Autodesk Inventor part; units mm, degrees
ref_plane "YZ Plane" through (0, 0, 0) normal (1, 0, 0) x (0, 1, 0)
ref_plane "XZ Plane" through (0, 0, 0) normal (0, 1, 0) x (-1, 0, 0)
ref_plane "XY Plane" through (0, 0, 0) normal (0, 0, 1) x (1, 0, 0)
sketch "Sketch1" plane through (0, 0, 0) normal (0, 1, 0) x (-1, 0, 0)
  line L0 (0, 0) -> (22.8, 0)
  line L1 (22.8, 0) -> (22.8, -12.6)
  line L2 (22.8, -12.6) -> (0, -12.6)
  line L3 (0, -12.6) -> (0, 0)
  dimension "d0" = 22.8
  dimension "d1" = 12.6
extrude "Extrusion1" add sketch "Sketch1" along normal blind 16
sketch "Sketch2" plane through (0, 16, 0) normal (0, 1, 0) x (1, 0, 0)
  line L0 (0, 0) -> (4.85, 0)
  line L1 (4.85, 0) -> (4.85, 12.6)
  line L2 (0, 12.6) -> (-22.8, 12.6)
  line L3 (4.85, 12.6) -> (-22.8, 12.6)
  line L4 (-22.8, 12.6) -> (-27.65, 12.6)
  line L5 (-27.65, 12.6) -> (-27.65, 0)
  line L6 (-27.65, 0) -> (4.85, 0)
  line L7 (-22.8, 0) -> (0, 0)
  dimension "d4" = 4.85
  dimension "d5" = 4.85
extrude "Extrusion2" add sketch "Sketch2" along normal blind 2
sketch "Sketch3" plane through (0, 18, 0) normal (0, 1, 0) x (1, 0, 0)
  line L0 (-27.65, 0) -> (-22.8, 0)
  line L1 (0, 0) -> (0, 12.6)
  line L2 (-22.8, 0) -> (0, 0)
  line L3 (0, 0) -> (0, 12.6)
  line L4 (0, 12.6) -> (-22.8, 12.6)
  line L5 (-22.8, 12.6) -> (-22.8, 0)
extrude "Extrusion3" add sketch "Sketch3" along normal blind 1
sketch "Sketch4" plane through (0, 18, 0) normal (0, 1, 0) x (1, 0, 0)
  line L0 (-27.65, 12.6) -> (-27.65, 0)
  circle A0 centre (-26.09, 6.3) radius 1
  circle A1 centre (3.29, 6.3) radius 1
  line L1 (4.85, 0) -> (4.85, 12.6)
  point P0 (0, 0)
  dimension "d11" = 1.56
  dimension "d12" = 2
  dimension "d13" = 2
  dimension "d14" = 1.56
extrude "Extrusion4" cut sketch "Sketch4" against normal through all
sketch "Sketch5" plane through (-27.65, 18, -12.6) normal (0, 1, 0) x (1, 0, 0)
  point P0 (27.65, -12.6)
sketch "Sketch6" plane through (-27.65, 18, -12.6) normal (0, 1, 0) x (1, 0, 0)
  line L0 (4.85, 0) -> (0, 0)
  line L1 (4.85, 0) -> (27.65, 0)
  line L2 (27.65, 0) -> (27.65, -12.6)
  line L3 (27.65, -12.6) -> (4.85, -12.6)
  line L4 (4.85, -12.6) -> (4.85, 0)
extrude "Extrusion5" add sketch "Sketch6" along normal blind 4.4
sketch "Sketch7" plane through (-27.65, 22.4, -12.6) normal (0, 1, 0) x (1, 0, 0)
  circle A0 centre (21.35, -6.3) radius 6.3
  line L0 (27.65, -12.6) -> (4.85, -12.6)
  line L1 (27.65, -12.6) -> (27.65, 0)
  circle A1 centre (14.1367, -6.3) radius 3
  dimension "d22" = 6.3
  dimension "d23" = 6
extrude "Extrusion6" add sketch "Sketch7" along normal blind 4.3 contours A0 A1 | A1 A0 picked at (24.082, -5.787) picked at (15.7711, -6.9546)
sketch "Sketch8" plane through (-27.65, 22.4, -12.6) normal (0, 1, 0) x (1, 0, 0)
  circle A0 centre (14.5284, -6.3) radius 3
  point P0 (27.65, -12.6)
  dimension "d26" = 6
extrude "Extrusion7" add sketch "Sketch8" along normal blind 4.3
sketch "Sketch9" plane through (-27.65, 26.7, -12.6) normal (0, 1, 0) x (1, 0, 0)
  arc A0 (15.6897, -9.0661) -> (15.6897, -3.5339) centre (21.35, -6.3) ccw
  circle A1 centre (21.35, -6.3) radius 2
  point P0 (27.65, -12.6)
  dimension "d29" = 4
extrude "Extrusion8" add sketch "Sketch9" along normal blind 4
properties part number "SG92R"
Verification items for the finished model (mm, model axes). A direction names the side the tool comes from. Round coordinates to 2 decimals unless told otherwise and drop trailing zeros. Write each loop counter-clockwise with the first axis right and the second up, starting at its lowest first coordinate (ties: lowest second). Pieces come first, ordered by that corner, then holes.
(1) Section check D-D (x = -10.5). Enter the section's corners in (y, z), plus the area to 3 significant figures.
Returned:
outline: (0, -12.6) - (22.4, -12.6) - (22.4, -11) - (26.7, -11) - (26.7, -1.6) - (22.4, -1.6) - (22.4, 0) - (0, 0) - close
area: 323 mm2
(2) Mould release check, pull along Z, two halves, no side actions. Record for faces 1 (the cylindrical face through (3.16, 17.01, -7.29)), 2 (the cylindrical face through (-25.136, 17.014, -6.6)), 3 (the flat face through (-1.5, 22.4, -11.3)), 4 (the cylindrical face through (-6.734, 28.672, -8.252)): pulls with the +Z half, pulls with the -Z half, needs draft (parallel to the pull), parting line crosses it, or undercut.
Returned:
face 1: undercut
face 2: undercut
face 3: needs draft
face 4: parting line crosses it
(3) Section check B-B (y = 17.5). Enter the section's corners in (x, z), plus the area to 3 significant figures.
Returned:
outline: (-27.65, -12.6) - (4.85, -12.6) - (4.85, 0) - (-27.65, 0) - close; hole circle Ø2 at (-26.09, -6.3); hole circle Ø2 at (3.29, -6.3)
area: 403 mm2
(4) Section check A-A (x = -26.09). Enter the section's corners in (y, z), plus the area to 3 significant figures.
Returned:
outline: (16, -12.6) - (18, -12.6) - (18, -7.3) - (16, -7.3) - close; (16, -5.3) - (18, -5.3) - (18, 0) - (16, 0) - close
area: 21.2 mm2
(5) Section check C-C (z = -10.5). Enter the section's corners in (x, y), plus the area to 3 significant figures.
Returned:
outline: (-27.65, 16) - (-22.8, 16) - (-22.8, 0) - (0, 0) - (0, 16) - (4.85, 16) - (4.85, 18) - (0, 18) - (0, 22.4) - (-1.6, 22.4) - (-1.6, 26.7) - (-11, 26.7) - (-11, 22.4) - (-22.8, 22.4) - (-22.8, 18) - (-27.65, 18) - close
area: 571 mm2
(6) Depth check by flat-ended pin: pin 1 Ø1.5 at (x, z) = (3, -7.5) entering from +Y; pin 2 Ø3 at (x, z) = (-3, -9.5) entering from +Y; pin 3 Ø3.5 at (y, z) = (20.5, -6) entering from -X. Enter the tip coordinate at first touch or a pass-through.
Returned:
pin 1: stops at y = 18
pin 2: stops at y = 26.7
pin 3: stops at x = -22.8
(7) Access from +Z, -Z, +X, -X, +Y, -Y to the whole of each face (thin tool, end or side, straight path). Record for faces 5 (the flat face through (2, 16, -6)), 6 (the flat face through (-22.8, 8, -6)), 7 (the cylindrical face through (-16.12, 24.52, -6.22)).
Returned:
face 5: +Z, -Z, +X, -Y
face 6: +Z, -Z, -X, -Y
face 7: +Y
(8) Material ranges on line 1 (X direction, y = 17.1, z = -6.3); line 2 (Z direction, x = -26.09, y = 17.1); line 3 (Y direction, x = 0.5, z = -8.5), recorded low to high.
Returned:
line 1: x = -27.65 to -27.09, -25.09 to 2.29, 4.29 to 4.85
line 2: z = -12.6 to -7.3, -5.3 to 0
line 3: y = 16 to 18
